Input: part model. Units: mm. Frame: model coordinates. Round coordinates to 2 decimals unless told otherwise and drop trailing zeros. Loops run counter-clockwise (first coordinate to the right, second up) from the corner with the lowest first, then second, coordinate; pieces in that order, holes last. Notation, with made-up numbers: M 19,89.25 L 68,89.25 A21 cw 68,121.25 Z; hole C 77,2.25 d3. An arc over 180 degrees is marked long. Use one line per item in the form item = value. Start each with the question number.
Q1. First-contact query: P1, Ø1.5, axis at y = -2.5, z = 4, coming from the +X side; P2, Ø1, axis at x = 19, z = 2, coming from the +Y side. Flat tips, straight axial feed; report the tip coordinate or a pass-through.
Q2. Ray query, line 1 along Y through (x, z) = (10, 1.2); line 2 along X through (y, z) = (0, 1.4); line 3 along Y through (x, z) = (7.5, 5.75). Return the intervals inside material, ascending.
Q3. Mould query, pull axis Y, two halves, no side actions, for faces 1 (the flat face through (10, 11, 6)), 2 (the cylindrical face through (0.46, -3, 2.79)). Classes: pulls with the +Y half, pulls with the -Y half, needs draft (parallel to the pull), parting line crosses it, or undercut.
Q4. Section query B-B, the plane y = 0. Output: boundary loops of the cut face in (x, z).
Q5. Section query A-A, the plane x = 10. Output: boundary loops of the cut face in (y, z), and give its area (3 significant figures).
Q6. Section query C-C, the plane z = 4.25. Output: boundary loops of the cut face in (x, y), and give its area (3 significant figures).
```python
from build123d import *


with BuildPart() as f1:
    # F0 (on Front) → F1 (revolve)
    with BuildSketch(Plane.XZ):
        with BuildLine():
            Line((-1.997872, 0), (0, 0))
            Line((0, 0), (0, 3))
            Line((0, 3), (-2, 3))
            ThreePointArc((-2, 3), (-2.867851, 2.039645), (-2.965851, 0.748969))
            ThreePointArc((-2.965851, 0.748969), (-2.609824, 0.209105), (-1.997872, 0))
        make_face()
        with BuildLine():
            Line((-2, 3), (0, 3))
            Line((0, 3), (0, 5.5))
            ThreePointArc((0, 5.5), (-0.146447, 5.853553), (-0.5, 6))
            Line((-0.5, 6), (-1.997872, 6))
            ThreePointArc((-1.997872, 6), (-2.609824, 5.790895), (-2.965851, 5.251031))
            ThreePointArc((-2.965851, 5.251031), (-2.867851, 3.960355), (-2, 3))
        make_face()
    revolve(axis=Axis((10, 0, 3), (0, 0, 1)))


solid = f1.part
```
Results found:
q1.P1 = 22.87
q1.P2 = 9.74
q2.line_1 = -13.03 to -10, 10 to 13.03
q2.line_2 = -3.02 to 0, 20 to 23.02
q2.line_3 = -12.41 to -9.75, 9.75 to 12.41
q3.face_1 = needs draft
q3.face_2 = undercut
q4.outline = M -2.97,0.75 A1 ccw -2,0 L 0,0 L 0,5.5 A0.5 ccw -0.5,6 L -2,6 A1 ccw -2.97,5.25 A2 ccw -2,3 A2 ccw Z; M 20,0 L 22,0 A1 ccw 22.97,0.75 A2 ccw 22,3 A2 ccw 22.97,5.25 A1 ccw 22,6 L 20.5,6 A0.5 ccw 20,5.5 Z
q5.outline = M -12.97,0.75 A1 ccw -12,0 L -10,0 L -10,5.5 A0.5 ccw -10.5,6 L -12,6 A1 ccw -12.97,5.25 A2 ccw -12,3 A2 ccw Z; M 10,0 L 12,0 A1 ccw 12.97,0.75 A2 ccw 12,3 A2 ccw 12.97,5.25 A1 ccw 12,6 L 10.5,6 A0.5 ccw 10,5.5 Z
q5.area = 33.2 mm²
q6.outline = C 10,0 d25.93; hole C 10,0 d20
q6.area = 214 mm²
